The model under review builds one solid part; all positions refer to its coordinate system, in mm. A direction names the side the tool comes from. Round coordinates to 2 decimals unless told otherwise and drop trailing zeros. Order: outer loops, then holes, each group sorted by start corner. A loop starts at its lowest first (then second) coordinate and runs counter-clockwise, first axis right, second up.
1) Consider section B-B (x = 0). Give the boundary of the cut face in (y, z), then the cut area to 3 significant figures.
2) To check wall thickness, follow L1, parallel to Y at x = 0, z = 1.15; L2, parallel to Z at x = 1.5, y = -27.5. State the ranges of each line that lie inside material, in increasing order.
3) Clearance check with flat-ended pins moving along their axes: P1, Ø1.8, axis at x = 30.5, z = 2.5, coming from the +Y side; P2, Ø1.8, axis at y = -0.5, z = 3, coming from the -X side; P3, Ø1.3, axis at y = -1, z = 2.5, coming from the +X side. State where each tip first meets the part, or that it passes through.
4) Consider section A-A (y = 0). Give the boundary of the cut face in (x, z), then the cut area to 3 significant figures.
5) Mouldability with a two-part tool opening along Y and no side actions: class faces 4 (the face through (23, -19, 3.22)), 5 (the face through (5.67, -31.95, 2.4)), 6 (the face through (27, 2, 1.6)) as pulls with the +Y half, pulls with the -Y half, needs draft (parallel to the pull), parting line crosses it, or undercut.
6) Machinability: for faces 1 (the face through (-24.58, -17.36, 2.4)), 2 (the face through (-30.48, -11.13, 2.4)), 3 (the face through (-21.05, -17.62, 2.4)), which of the approach directions +Z, -Z, +X, -X, +Y, -Y give a long, thin tool a straight path to every point of the face, cutting with its end or side? Answer none if there is none.
7) Consider section D-D (y = 9.5). Give the boundary of the cut face in (x, z).
8) Consider section C-C (z = 2.1). Give the number of separate pieces and of enclosed holes in the cut face, then the cut area to 3 significant figures.
Solid Edge part; units mm, degrees
sketch "Sketch1" plane through (0, 0, 0) normal (0, -1, 0) x (1, 0, 0)
  line L0 (-33, 1.6) -> (-33, 0)
  line L1 (-33, 0) -> (-26.9, 0)
  line L2 (-26.9, 0) -> (-26.9, 1.6)
  line L3 (-26.9, 1.6) -> (-33, 1.6)
  dimension "D1" = 33
revolve "RevolvedProtrusion1" add sketch "Sketch1" angle 360 about axis through (0, 0, 0) along (0, 0, 1)
sketch "Sketch2" plane through (0, 0, 1.6) normal (0, 0, 1) x (1, 0, 0)
  line L0 (-32.45, 2.5) -> (-27.45, 2.5)
  line L1 (-27.45, 2.5) -> (-27.45, -2.5)
  line L2 (-27.45, -2.5) -> (-32.45, -2.5)
  line L3 (-32.45, -2.5) -> (-32.45, 2.5)
  dimension "D1" = 32.45
  dimension "D2" = 32.45
extrude "Protrusion1" add sketch "Sketch2" along normal blind 1.62
pattern_circular "Pattern1" count 18 over 360 about axis through (0, 0, 1.6) along (0, 0, 1) of "Protrusion1"
Answer below:
1. outline: (-33, 0) - (-26.9, 0) - (-26.9, 1.6) - (-33, 1.6) - close; (26.9, 0) - (33, 0) - (33, 1.6) - (26.9, 1.6) - close
1. area: 19.5 mm2
2. L1: y = -33 to -26.9, 26.9 to 33
2. L2: z = 0 to 1.6
3. P1: stops at y = 13.45
3. P2: stops at x = -32.45
3. P3: stops at x = 32.45
4. outline: (-33, 0) - (-26.9, 0) - (-26.9, 1.6) - (-27.45, 1.6) - (-27.45, 3.22) - (-32.45, 3.22) - (-32.45, 1.6) - (-33, 1.6) - close; (26.9, 0) - (33, 0) - (33, 1.6) - (32.45, 1.6) - (32.45, 3.22) - (27.45, 3.22) - (27.45, 1.6) - (26.9, 1.6) - close
4. area: 35.7 mm2
5. face 4: needs draft
5. face 5: pulls with the -Y half
5. face 6: undercut
6. face 1: +Z, -X
6. face 2: +Z, -X, -Y
6. face 3: +Z
7. outline: (-31.6, 0) - (-25.17, 0) - (-25.17, 1.6) - (-25.75, 1.6) - (-25.75, 3.22) - (-31.07, 3.22) - (-31.07, 1.6) - (-31.6, 1.6) - close; (25.17, 0) - (31.6, 0) - (31.6, 1.6) - (31.07, 1.6) - (31.07, 3.22) - (25.75, 3.22) - (25.75, 1.6) - (25.17, 1.6) - close
8. separate pieces: 18
8. enclosed holes: 0
8. area: 450 mm2
